Autodesk Fusion 360 part; units mm, degrees
sketch "Skizze1" plane through (0, 0, 0) normal (0, 0, 1) x (1, 0, 0)
  line L0 (0, 0) -> (107, 0)
  line L1 (107, 0) -> (107, 69.5)
  line L2 (107, 69.5) -> (0, 69.5)
  line L3 (0, 69.5) -> (0, 0)
  dimension "d1" = 107
  dimension "d2" = 69.5
extrude "Extrusion1" add sketch "Skizze1" along normal blind 3
sketch "Skizze2" plane through (0, 0, 0) normal (0, 0, -1) x (1, 0, 0)
  line L0 (0, 0) -> (0, -69.5)
  line L1 (0, -69.5) -> (107, -69.5)
  line L2 (107, -69.5) -> (107, 0)
  line L3 (107, 0) -> (0, 0)
  line L4 (0, 0) -> (7, 0)
  line L5 (7, 0) -> (7, -7)
  line L6 (7, -7) -> (0, -7)
  line L7 (0, -7) -> (0, 0)
  line L8 (107, 0) -> (100, 0)
  line L9 (100, 0) -> (100, -7)
  line L10 (100, -7) -> (107, -7)
  line L11 (107, -7) -> (107, 0)
  line L12 (107, -69.5) -> (100, -69.5)
  line L13 (100, -69.5) -> (100, -62.5)
  line L14 (100, -62.5) -> (107, -62.5)
  line L15 (107, -62.5) -> (107, -69.5)
  line L16 (0, -69.5) -> (7, -69.5)
  line L17 (7, -69.5) -> (7, -62.5)
  line L18 (7, -62.5) -> (0, -62.5)
  line L19 (0, -62.5) -> (0, -69.5)
  circle A0 centre (3.5, -66) radius 2.65
  circle A1 centre (103.5, -66) radius 2.65
  circle A2 centre (103.5, -3.5) radius 2.65
  circle A3 centre (3.5, -3.5) radius 2.65
  dimension "d5" = 7
  dimension "d6" = 7
  dimension "d7" = 7
  dimension "d8" = 7
  dimension "d9" = 7
  dimension "d10" = 7
  dimension "d11" = 7
  dimension "d12" = 7
  dimension "d13" = 5.3
  dimension "d14" = 5.3
  dimension "d15" = 5.3
  dimension "d16" = 5.3
  dimension "d17" = 3.5
  dimension "d18" = 3.5
  dimension "d19" = 3.5
  dimension "d20" = 3.5
  dimension "d21" = 3.5
  dimension "d22" = 3.5
  dimension "d23" = 3.5
  dimension "d24" = 3.5
extrude "Extrusion2" cut sketch "Skizze2" against normal blind 1.2 contours A0 | A1 | A2 | A3
fillet "Abrundung1" radius 2 4 edges at (0, 0, 1.5) (107, 0, 1.5) (107, 69.5, 1.5) (0, 69.5, 1.5)
sketch "Skizze3" plane through (0, 0, 3) normal (0, 0, 1) x (-1, 0, 0)
  arc A0 (-2, -69.5) -> (0, -67.5) centre (-2, -67.5) ccw
  line L0 (0, -67.5) -> (0, -2)
  arc A1 (0, -2) -> (-2, 0) centre (-2, -2) ccw
  line L1 (-2, 0) -> (-105, 0)
  arc A2 (-105, 0) -> (-107, -2) centre (-105, -2) ccw
  line L2 (-107, -2) -> (-107, -67.5)
  arc A3 (-107, -67.5) -> (-105, -69.5) centre (-105, -67.5) ccw
  line L3 (-105, -69.5) -> (-2, -69.5)
  line L4 (-33, -61.5) -> (-74, -61.5)
  line L5 (-74, -61.5) -> (-74, -8)
  line L6 (-74, -8) -> (-33, -8)
  line L7 (-33, -8) -> (-33, -61.5)
  circle A4 centre (-33, -34.75) radius 15
  circle A5 centre (-74, -34.75) radius 15
  dimension "d29" = 41
  dimension "d30" = 53.5
  dimension "d31" = 33
  dimension "d32" = 8
  dimension "d33" = 30
  dimension "d34" = 30
extrude "Extrusion3" cut sketch "Skizze3" against normal blind 2 contours L4 L5 L6 L7 A4 A5 | L7 A4 | L7 A4 | L5 A5 | L5 A5
equation "d31 = ( ( 74 / 2 ) * 1 mm ) - 4 mm"
For this review, take the finished solid that the model builds, in its own axes (mm). A direction names the side the tool comes from. Round coordinates to 2 decimals unless told otherwise and drop trailing zeros. Write each loop counter-clockwise with the first axis right and the second up, starting at its lowest first coordinate (ties: lowest second). Pieces come first, ordered by that corner, then holes. Notation, with made-up numbers: (-14, 48) - (0, 48) arc R17 ccw to (0, 54) - close; hole circle Ø3 at (50, 20). An arc over 180 degrees is marked (long way). Answer as a JSON object with one key per item and string values.
1. To check wall thickness, follow line 1 along X through (y, z) = (66, 0.4); line 2 along Y through (x, z) = (3.5, 0.5); line 3 along X through (y, z) = (35, 1.65). State the ranges of each line that lie inside material, in increasing order.
Response values:
{"line 1": "x = 0 to 0.85, 6.15 to 100.85, 106.15 to 107", "line 2": "y = 0 to 0.85, 6.15 to 63.35, 68.65 to 69.5", "line 3": "x = 0 to 18, 89 to 107"}
2. For pin 1 Ø2.5 at (x, y) = (104, 3) entering from -Z; pin 2 Ø4 at (x, y) = (104.5, 65) entering from -Z, all flat-tipped, find the tip position at first contact; note any pin that passes through.
Response values:
{"pin 1": "stops at z = 1.2", "pin 2": "stops at z = 0"}
3. Draft analysis for pull direction X (two halves, no side actions). For faces 1 (the face through (103, 66, 1.2)), 2 (the face through (53, 35, 0)), 3 (the face through (0.57, 0.6, 1.52)), state which applies: +X half, -X half, draft (parallel to the pull), parting line (faces both ways), or undercut.
Response values:
{"face 1": "undercut", "face 2": "draft", "face 3": "-X half"}
4. Tool access review of faces 4 (the face through (0.6, 68.93, 1.52)), 5 (the face through (18.004, 35.08, 2.014)), 6 (the face through (2.93, 68.59, 0.59)): name each direction out of +Z, -Z, +X, -X, +Y, -Y from which nothing blocks a thin tool from reaching the whole face with its end or side.
Response values:
{"face 4": "+Z, -Z, -X, +Y", "face 5": "+Z", "face 6": "-Z"}
5. We need section D-D on x = 3.5. Give the boundary of the cut face in (y, z), then the cut area to 3 significant figures.
Response values:
{"outline": "(0, 0) - (0.85, 0) - (0.85, 1.2) - (6.15, 1.2) - (6.15, 0) - (63.35, 0) - (63.35, 1.2) - (68.65, 1.2) - (68.65, 0) - (69.5, 0) - (69.5, 3) - (0, 3) - close", "area": "196 mm2"}
6. We need section C-C on y = 34.75. Give the boundary of the cut face in (x, z), then the cut area to 3 significant figures.
Response values:
{"outline": "(0, 0) - (107, 0) - (107, 3) - (89, 3) - (89, 1) - (18, 1) - (18, 3) - (0, 3) - close", "area": "179 mm2"}
7. We need section B-B on x = 24. Give the boundary of the cut face in (y, z).
Response values:
{"outline": "(0, 0) - (69.5, 0) - (69.5, 3) - (46.75, 3) - (46.75, 1) - (22.75, 1) - (22.75, 3) - (0, 3) - close"}
8. We need section A-A on z = 1.95. Give the boundary of the cut face in (x, y), then the cut area to 3 significant figures.
Response values:
{"outline": "(0, 2) arc R2 ccw to (2, 0) - (105, 0) arc R2 ccw to (107, 2) - (107, 67.5) arc R2 ccw to (105, 69.5) - (2, 69.5) arc R2 ccw to (0, 67.5) - close; hole (33, 8) - (74, 8) - (74, 19.75) arc R15 ccw to (74, 49.75) - (74, 61.5) - (33, 61.5) - (33, 49.75) arc R15 ccw to (33, 19.75) - close", "area": "4,530 mm2"}
